Model file for the job. Use its own axes, mm. A direction names the side the tool comes from. Coordinates: 2 decimals unless noted, no trailing zeros. Write each loop counter-clockwise with the first axis right and the second up, starting at its lowest first coordinate (ties: lowest second). Pieces come first, ordered by that corner, then holes. Notation, with made-up numbers: (9.5, 51.5) - (55.5, 51.5) arc R22 cw to (55.5, 79.5) - close; hole circle Ø8 at (53, 49). An arc over 180 degrees is marked (long way). Put each result on its own line as item: value. Start each with the question number.
1. Which spindle directions (+Z, -Z, +X, -X, +Y, -Y) get a long thin tool onto all of the face, cutting with end or side? Do faces 1 (the face through (25, 3, 7)), 2 (the face through (34.7, 140, 12.4)), 3 (the face through (35, 0, 13)), 4 (the face through (35, 121, 14)), 5 (the face through (57, 6, 7)). Say none if no direction does.
2. Drill centre lines: L1, parallel to Y at x = 50, z = 2.75; L2, parallel to Y at x = 20, z = 4.25; L3, parallel to Y at x = 51.5, z = 7.5. Where is each one in solid material? Low to high. Write a range as from..to.
3. Saw through at B-B, the plane z = 8.5. Give the number of separate pieces and of enclosed holes in the cut face, plus the area to 3 significant figures.
4. Pull direction X, two halves, no side cores. Call faces 6 (the face through (25, 131, 7)), 7 (the face through (4.28, 135.49, 7.6)), 8 (the face through (45, 131, 7)), 9 (the face through (12, 18.2, 7)): released by +X, released by -X, zero draft, split by the parting line, or undercut.
5. Saw through at A-A, the plane y = 72. Write the cut outline in (x, z).
6. Saw through at D-D, the plane y = 99.5. Write the cut outline in (x, z).
7. Drop flat-ended pins along their axis: P1, Ø1.2, axis at x = 61.5, y = 34.5, coming from the +Z side; P2, Ø1.6, axis at x = 27.5, z = 15.5, coming from the +Y side; P3, Ø8, axis at y = 131, z = 7.5, coming from the +X side. Give the stop position or say it passes through.
8. Saw through at C-C, the plane x = 39. Write the cut outline in (y, z).
```python
from build123d import *

# Parameters (mm, degrees)
BOX_W           = 70
BOX_H           = 140
BOX_DEPTH       = 16
SKETCH_R        = 1
POCKET_DEPTH    = 20
SKETCH001_W     = 12.2
SKETCH001_H     = 10.2
SKETCH001_W_2   = 42
SKETCH001_H_2   = 5.1
POCKET001_DEPTH = 75
SKETCH002_W     = 20
SKETCH002_H     = 10.2
POCKET002_DEPTH = 140
SKETCH003_W     = 34
SKETCH003_H     = 38.5
SKETCH003_W_2   = 60
SKETCH003_H_2   = 90
POCKET003_DEPTH = 2
SKETCH004_W     = 4
SKETCH004_H     = 4
POCKET004_DEPTH = 80
FILLET_R        = 15
FILLET001_R     = 1


with BuildPart() as part:
    # Box → Box (new body)
    with BuildSketch(Plane.XY):
        with Locations((35, 70)):
            Rectangle(BOX_W, BOX_H)
    extrude(amount=BOX_DEPTH)

    # Sketch (on Face6 of BaseFeature) → Pocket (cut)
    with BuildSketch(Plane.XY.offset(16)):
        with Locations((3, 3)):
            Circle(SKETCH_R)
        with Locations((67, 3)):
            Circle(SKETCH_R)
        with Locations((3, 87)):
            Circle(SKETCH_R)
        with Locations((67, 87)):
            Circle(SKETCH_R)
        with Locations((21.5, 137)):
            Circle(SKETCH_R)
        with Locations((48.5, 137)):
            Circle(SKETCH_R)
        with Locations((21.5, 106)):
            Circle(SKETCH_R)
        with Locations((48.5, 106)):
            Circle(SKETCH_R)
    extrude(amount=-POCKET_DEPTH, mode=Mode.SUBTRACT)

    # Sketch001 → Pocket001 (cut)
    with BuildSketch(Plane.YZ):
        with Locations((12.1, 7.1)):
            Rectangle(SKETCH001_W, SKETCH001_H)
        with Locations((116.1, 7.1)):
            Rectangle(SKETCH001_W, SKETCH001_H)
        with Locations((61, 4.55)):
            Rectangle(SKETCH001_W_2, SKETCH001_H_2)
    extrude(amount=POCKET001_DEPTH, mode=Mode.SUBTRACT)

    # Sketch002 → Pocket002 (cut)
    with BuildSketch(Plane.XZ):
        with Locations((35, 7.1)):
            Rectangle(SKETCH002_W, SKETCH002_H)
    extrude(amount=-POCKET002_DEPTH, mode=Mode.SUBTRACT)

    # Sketch003 (on Face3 of Pocket002) → Pocket003 (cut)
    with BuildSketch(Plane.XY.offset(16)):
        with Locations((35, 120.75)):
            Rectangle(SKETCH003_W, SKETCH003_H)
        with Locations((35, 43)):
            Rectangle(SKETCH003_W_2, SKETCH003_H_2)
    extrude(amount=-POCKET003_DEPTH, mode=Mode.SUBTRACT)

    # Sketch004 (on Face18 of Pocket003) → Pocket004 (cut)
    with BuildSketch(Plane.YZ.offset(70)):
        with Locations((35, 5)):
            Rectangle(SKETCH004_W, SKETCH004_H)
    extrude(amount=-POCKET004_DEPTH, mode=Mode.SUBTRACT)

    # Fillet
    fillet_edges = [part.edges().sort_by_distance(p)[0] for p in [
        (0, 140, 8),
        (70, 140, 8),
    ]]
    fillet(fillet_edges, radius=FILLET_R)

    # Fillet001
    fillet001_edges = [part.edges().sort_by_distance(p)[0] for p in [
        (70, 0, 8),
        (0, 0, 8),
        (70, 62.5, 16),
        (0, 62.5, 16),
        (65.606602, 135.606602, 16),
        (53.5, 140, 16),
        (16.5, 140, 16),
        (4.393398, 135.606602, 16),
    ]]
    fillet(fillet001_edges, radius=FILLET001_R)


solid = part.part
```
Final values:
1. face 1: +Y, -Y
1. face 2: +Z, -Z, +X, -X, +Y
1. face 3: +Z, -Z, +X, -X, -Y
1. face 4: +Z, +Y
1. face 5: +X, -X
2. L1: y = 0..6, 18.2..40, 82..110, 122.2..140
2. L2: y = 0..6, 18.2..33, 37..40, 82..110, 122.2..140
2. L3: y = 0..6, 18.2..110, 122.2..140
3. separate pieces: 6
3. enclosed holes: 8
3. area: 5,660 mm²
4. face 6: undercut
4. face 7: released by -X
4. face 8: undercut
4. face 9: zero draft
5. outline: (0, 0) - (70, 0) - (70, 2) - (0, 2) - close; (0, 7.1) - (25, 7.1) - (25, 12.2) - (45, 12.2) - (45, 7.1) - (70, 7.1) - (70, 15) arc R1 ccw to (69, 16) - (65, 16) - (65, 14) - (5, 14) - (5, 16) - (1, 16) arc R1 ccw to (0, 15) - close
6. outline: (0, 0) - (70, 0) - (70, 15) arc R1 ccw to (69, 16) - (1, 16) arc R1 ccw to (0, 15) - close; hole (25, 2) - (45, 2) - (45, 12.2) - (25, 12.2) - close
7. P1: stops at z = 14
7. P2: stops at y = 101.5
7. P3: stops at x = 69.87
8. outline: (0, 0) - (140, 0) - (140, 2) - (0, 2) - close; (0, 12.2) - (140, 12.2) - (140, 14) - (101.5, 14) - (101.5, 16) - (88, 16) - (88, 14) - (0, 14) - close
